Source: three-view drawing plus pictorial views. Frame: mm from the lowest corner of the part. A direction names the side the tool comes from. Coordinates: 2 decimals unless noted, no trailing zeros. Loops run counter-clockwise (first coordinate to the right, second up) from the corner with the lowest first, then second, coordinate; pieces in that order, holes last. Notation, with made-up numbers: M 11,0 L 20,0 A35 ccw 20,34 Z; hole C 9.5,33.5 d2. An arc over 180 degrees is marked long. Use a Markdown table: item, result. Add a question column.
1. Section C-C on x = 21.75. Output: boundary loops of the cut face in (y, z).
2. Section A-A on z = 12.5. Output: boundary loops of the cut face in (x, y).
3. Set-up query: the marked faces 1, 2 and 3. Return all of +Z, -Z, +X, -X, +Y, -Y with unobstructed straight access to the full face (end or side cutting, diameter ignored); none if empty.
4. Section B-B on y = 12.5. Output: boundary loops of the cut face in (x, z).
5. Line query: L1, parallel to X at y = 6.25, z = 6.5; L2, parallel to X at y = 11.5, z = 13; L3, parallel to Z at x = 1.75, y = 17.25. Output: solid intervals per line, ascending. Write a range as [from, to].
6. Pin query (flat end, axial travel): pin 1 (6 mm diameter, centred on x = 20.5, y = 12.5, fed in from -Z); pin 2 (1.5 mm diameter, centred on x = 5.5, z = 18.5, fed in from -Y); pin 3 (1 mm diameter, centred on y = 12.5, z = 12.5, fed in from -X); pin 4 (0.9 mm diameter, centred on x = 1, y = 13, fed in from +Z). Return the tip coordinate at first contact, or that it passes through.
7. Draft query along Z for the marked faces 4, 5 and 6. Return one class per face: +Z half, -Z half, draft (parallel to the pull), parting line (faces both ways), or undercut.
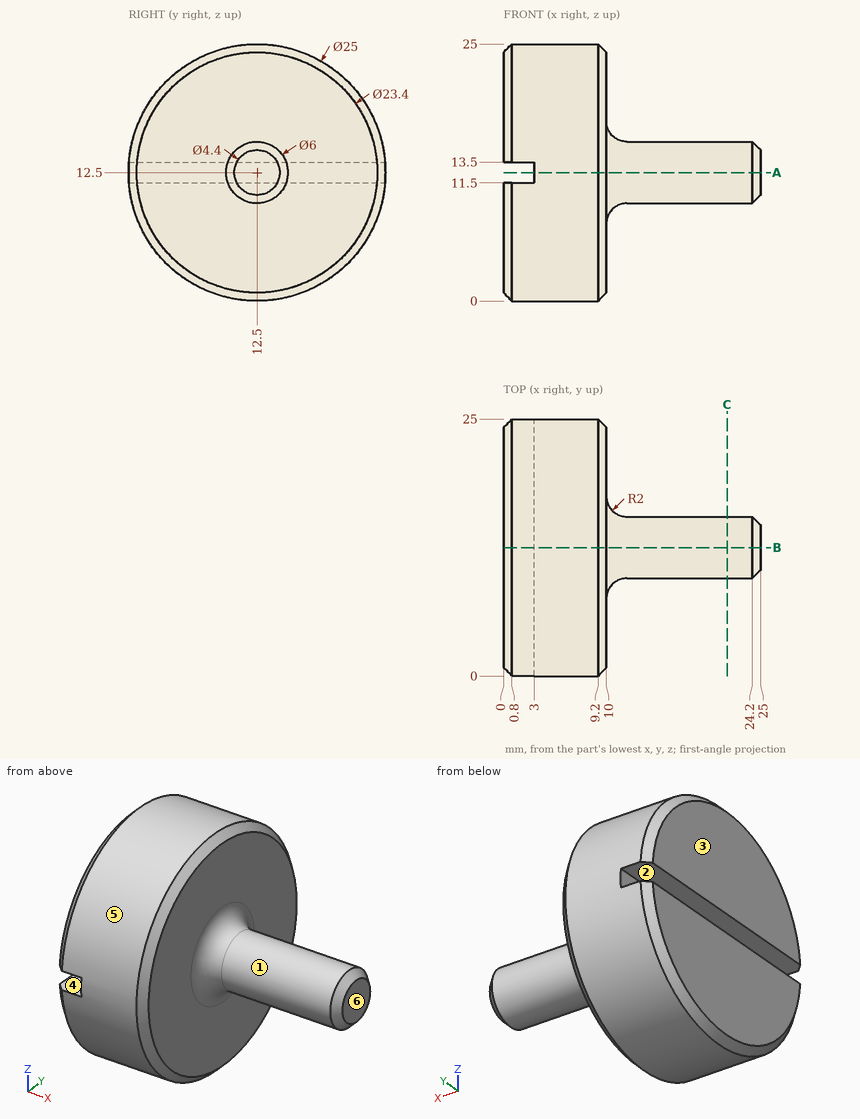
Answers below:
| question | item | result |
|---|---|---|
| 1 | outline | C 12.5,12.5 d6 |
| 2 | outline | M 3,0 L 9.2,0 L 10,0.8 L 10,7.5 A2 cw 12,9.5 L 24.2,9.5 L 25,10.3 L 25,14.7 L 24.2,15.5 L 12,15.5 A2 cw 10,17.5 L 10,24.2 L 9.2,25 L 3,25 Z |
| 3 | face 1 | +X |
| 3 | face 2 | -X, +Y, -Y |
| 3 | face 3 | +Z, -Z, -X, +Y, -Y |
| 4 | outline | M 0,0.8 L 0.8,0 L 9.2,0 L 10,0.8 L 10,7.5 A2 cw 12,9.5 L 24.2,9.5 L 25,10.3 L 25,14.7 L 24.2,15.5 L 12,15.5 A2 cw 10,17.5 L 10,24.2 L 9.2,25 L 0.8,25 L 0,24.2 L 0,13.5 L 3,13.5 L 3,11.5 L 0,11.5 Z |
| 5 | L1 | x = [0, 10] |
| 5 | L2 | x = [3, 25] |
| 5 | L3 | z = [0.94, 11.5], [13.5, 24.06] |
| 6 | pin 1 | stops at z = 9.5 |
| 6 | pin 2 | stops at y = 1.16 |
| 6 | pin 3 | stops at x = 3 |
| 6 | pin 4 | stops at z = 25 |
| 7 | face 4 | undercut |
| 7 | face 5 | parting line |
| 7 | face 6 | draft |
